Solid Edge part; units mm, degrees
sketch "Sketch1" plane through (0, 0, 0) normal (0, 0, 1) x (1, 0, 0)
  line L0 (400, 0) -> (0, 0)
  line L1 (0, 0) -> (0, 400)
  line L2 (0, 400) -> (400, 400)
  line L3 (400, 400) -> (400, 0)
extrude "Protrusion1" add sketch "Sketch1" along normal blind 15
sketch "Sketch2" plane through (200, 200, 15) normal (0, 0, 1) x (1, 0, 0)
  circle A0 centre (-170, 180) radius 5
extrude "VaciadoExtruido_1" cut sketch "Sketch2" against normal blind 15
sketch "Sketch3" plane through (200, 200, 15) normal (0, 0, 1) x (1, 0, 0)
  circle A0 centre (170, -180) radius 5
extrude "VaciadoExtruido_7" cut sketch "Sketch3" against normal blind 15
sketch "Sketch4" plane through (200, 200, 15) normal (0, 0, 1) x (1, 0, 0)
  circle A0 centre (-170, -180) radius 5
extrude "VaciadoExtruido_10" cut sketch "Sketch4" against normal blind 15
sketch "Sketch5" plane through (200, 200, 15) normal (0, 0, 1) x (1, 0, 0)
  circle A0 centre (170, 180) radius 5
extrude "VaciadoExtruido_13" cut sketch "Sketch5" against normal blind 15
sketch "Sketch6" plane through (200, 200, 15) normal (0, 0, 1) x (1, 0, 0)
  circle A0 centre (-182, 168) radius 2
extrude "VaciadoExtruido_14" cut sketch "Sketch6" against normal blind 15
sketch "Sketch7" plane through (200, 200, 15) normal (0, 0, 1) x (1, 0, 0)
  circle A0 centre (182, -192) radius 2
extrude "VaciadoExtruido_15" cut sketch "Sketch7" against normal blind 15
sketch "Sketch8" plane through (200, 200, 15) normal (0, 0, 1) x (1, 0, 0)
  circle A0 centre (182, -168) radius 2
extrude "VaciadoExtruido_16" cut sketch "Sketch8" against normal blind 15
sketch "Sketch9" plane through (200, 200, 15) normal (0, 0, 1) x (1, 0, 0)
  circle A0 centre (158, -192) radius 2
extrude "VaciadoExtruido_17" cut sketch "Sketch9" against normal blind 15
sketch "Sketch10" plane through (200, 200, 15) normal (0, 0, 1) x (1, 0, 0)
  circle A0 centre (158, -168) radius 2
extrude "VaciadoExtruido_18" cut sketch "Sketch10" against normal blind 15
sketch "Sketch11" plane through (200, 200, 15) normal (0, 0, 1) x (1, 0, 0)
  circle A0 centre (-158, -192) radius 2
extrude "VaciadoExtruido_19" cut sketch "Sketch11" against normal blind 15
sketch "Sketch12" plane through (200, 200, 15) normal (0, 0, 1) x (1, 0, 0)
  circle A0 centre (-182, -192) radius 2
extrude "VaciadoExtruido_20" cut sketch "Sketch12" against normal blind 15
sketch "Sketch13" plane through (200, 200, 15) normal (0, 0, 1) x (1, 0, 0)
  circle A0 centre (-182, -168) radius 2
extrude "VaciadoExtruido_21" cut sketch "Sketch13" against normal blind 15
sketch "Sketch14" plane through (200, 200, 15) normal (0, 0, 1) x (1, 0, 0)
  circle A0 centre (-158, -168) radius 2
extrude "VaciadoExtruido_22" cut sketch "Sketch14" against normal blind 15
sketch "Sketch15" plane through (200, 200, 15) normal (0, 0, 1) x (1, 0, 0)
  circle A0 centre (182, 168) radius 2
extrude "VaciadoExtruido_23" cut sketch "Sketch15" against normal blind 15
sketch "Sketch16" plane through (200, 200, 15) normal (0, 0, 1) x (1, 0, 0)
  circle A0 centre (158, 168) radius 2
extrude "VaciadoExtruido_24" cut sketch "Sketch16" against normal blind 15
sketch "Sketch17" plane through (200, 200, 15) normal (0, 0, 1) x (1, 0, 0)
  circle A0 centre (158, 192) radius 2
extrude "VaciadoExtruido_25" cut sketch "Sketch17" against normal blind 15
sketch "Sketch18" plane through (200, 200, 15) normal (0, 0, 1) x (1, 0, 0)
  circle A0 centre (182, 192) radius 2
extrude "VaciadoExtruido_26" cut sketch "Sketch18" against normal blind 15
sketch "Sketch19" plane through (200, 200, 15) normal (0, 0, 1) x (1, 0, 0)
  circle A0 centre (-158, 168) radius 2
extrude "VaciadoExtruido_27" cut sketch "Sketch19" against normal blind 15
sketch "Sketch20" plane through (200, 200, 15) normal (0, 0, 1) x (1, 0, 0)
  circle A0 centre (-158, 192) radius 2
extrude "VaciadoExtruido_29" cut sketch "Sketch20" against normal blind 15
sketch "Sketch21" plane through (200, 200, 15) normal (0, 0, 1) x (1, 0, 0)
  circle A0 centre (-182, 192) radius 2
extrude "VaciadoExtruido_30" cut sketch "Sketch21" against normal blind 15
sketch "Sketch22" plane through (200, 200, 15) normal (0, 0, 1) x (1, 0, 0)
  circle A0 centre (-80, -170) radius 7.5
extrude "VaciadoExtruido_32" cut sketch "Sketch22" against normal blind 15
sketch "Sketch23" plane through (200, 200, 15) normal (0, 0, 1) x (1, 0, 0)
  circle A0 centre (80, -170) radius 7.5
extrude "VaciadoExtruido_33" cut sketch "Sketch23" against normal blind 15
sketch "Sketch24" plane through (200, 200, 15) normal (0, 0, 1) x (0, 1, 0)
  circle A0 centre (0, 90) radius 4.5
extrude "VaciadoExtruido_34" cut sketch "Sketch24" against normal blind 15
sketch "Sketch25" plane through (200, 200, 15) normal (0, 0, 1) x (0, 1, 0)
  circle A0 centre (0, -90) radius 4.5
extrude "VaciadoExtruido_35" cut sketch "Sketch25" against normal blind 15
sketch "Sketch26" plane through (200, 200, 15) normal (0, 0, 1) x (0, 1, 0)
  circle A0 centre (-155, 60) radius 2
extrude "VaciadoExtruido_36" cut sketch "Sketch26" against normal blind 15
sketch "Sketch27" plane through (200, 200, 15) normal (0, 0, 1) x (0, 1, 0)
  circle A0 centre (-185, 60) radius 2
extrude "VaciadoExtruido_37" cut sketch "Sketch27" against normal blind 15
sketch "Sketch28" plane through (200, 200, 15) normal (0, 0, 1) x (0, 1, 0)
  circle A0 centre (-185, 100) radius 2
extrude "VaciadoExtruido_38" cut sketch "Sketch28" against normal blind 15
sketch "Sketch29" plane through (200, 200, 15) normal (0, 0, 1) x (0, 1, 0)
  circle A0 centre (-155, 100) radius 2
extrude "VaciadoExtruido_39" cut sketch "Sketch29" against normal blind 15
sketch "Sketch30" plane through (200, 200, 15) normal (0, 0, 1) x (0, 1, 0)
  circle A0 centre (-155, -100) radius 2
extrude "VaciadoExtruido_40" cut sketch "Sketch30" against normal blind 15
sketch "Sketch31" plane through (200, 200, 15) normal (0, 0, 1) x (0, 1, 0)
  circle A0 centre (-185, -100) radius 2
extrude "VaciadoExtruido_41" cut sketch "Sketch31" against normal blind 15
sketch "Sketch32" plane through (200, 200, 15) normal (0, 0, 1) x (0, 1, 0)
  circle A0 centre (-155, -60) radius 2
extrude "VaciadoExtruido_42" cut sketch "Sketch32" against normal blind 15
sketch "Sketch33" plane through (200, 200, 15) normal (0, 0, 1) x (0, 1, 0)
  circle A0 centre (-185, -60) radius 2
extrude "VaciadoExtruido_43" cut sketch "Sketch33" against normal blind 15
sketch "Sketch34" plane through (200, 200, 15) normal (0, 0, 1) x (0, 1, 0)
  circle A0 centre (-9.9999, -89.9472) radius 2
extrude "VaciadoExtruido_44" cut sketch "Sketch34" against normal blind 15
sketch "Sketch35" plane through (200, 200, 15) normal (0, 0, 1) x (0, 1, 0)
  circle A0 centre (0.0102, -100) radius 2
extrude "VaciadoExtruido_45" cut sketch "Sketch35" against normal blind 15
sketch "Sketch36" plane through (200, 200, 15) normal (0, 0, 1) x (0, 1, 0)
  circle A0 centre (9.9999, -89.9472) radius 2
extrude "VaciadoExtruido_46" cut sketch "Sketch36" against normal blind 15
sketch "Sketch37" plane through (200, 200, 15) normal (0, 0, 1) x (0, 1, 0)
  circle A0 centre (0, -80) radius 2
extrude "VaciadoExtruido_47" cut sketch "Sketch37" against normal blind 15
sketch "Sketch38" plane through (200, 200, 15) normal (0, 0, 1) x (0, 1, 0)
  circle A0 centre (0, 100) radius 2
extrude "VaciadoExtruido_48" cut sketch "Sketch38" against normal blind 15
sketch "Sketch39" plane through (200, 200, 15) normal (0, 0, 1) x (0, 1, 0)
  circle A0 centre (-10, 90) radius 2
extrude "VaciadoExtruido_49" cut sketch "Sketch39" against normal blind 15
sketch "Sketch40" plane through (200, 200, 15) normal (0, 0, 1) x (0, 1, 0)
  circle A0 centre (0, 80) radius 2
extrude "VaciadoExtruido_50" cut sketch "Sketch40" against normal blind 15
sketch "Sketch41" plane through (200, 200, 15) normal (0, 0, 1) x (0, 1, 0)
  circle A0 centre (10, 90) radius 2
extrude "VaciadoExtruido_51" cut sketch "Sketch41" against normal blind 15
Read the model definition and answer for the solid it produces. Units are mm, in the model's axes. Give positions to 0.01 mm unless a question says otherwise; leave off trailing zeros. Loops run counter-clockwise (first coordinate to the right, second up) from the corner with the lowest first, then second, coordinate; pieces in that order, holes last. Notation, with made-up numbers: (51, 1.5) - (100, 1.5) arc R23 ccw to (100, 15.5) - close; hole circle Ø5 at (64, 65.5). An arc over 180 degrees is marked (long way). Answer as CSV lines item,"result". Start each with the question number.
1) Determine the mould class of faces 1 (the face through (203, 0, 7)), 2 (the face through (29.349, 384.957, 7.605)), 3 (the face through (197, 400, 7)) for opening direction Y: released by +Y, released by -Y, zero draft, split by the parting line, or undercut.
2) Find section A-A (x = 370). Write down the section's boundary in (y, z).
3) Straight lines are drawn through the part: L1, parallel to X at y = 380, z = 4.5; L2, parallel to Y at x = 280, z = 10.5; L3, parallel to X at y = 381, z = 13.75. For each, find the intervals that lie inside material, in ascending order. Write a range as from..to.
Findings below:
1,face 1,"released by -Y"
1,face 2,"undercut"
1,face 3,"released by +Y"
2,outline,"(0, 0) - (15, 0) - (15, 15) - (0, 15) - close; (25, 0) - (375, 0) - (375, 15) - (25, 15) - close; (385, 0) - (400, 0) - (400, 15) - (385, 15) - close"
3,L1,"0..25, 35..365, 375..400"
3,L2,"0..22.5, 37.5..198, 202..400"
3,L3,"0..25.1, 34.9..365.1, 374.9..400"
